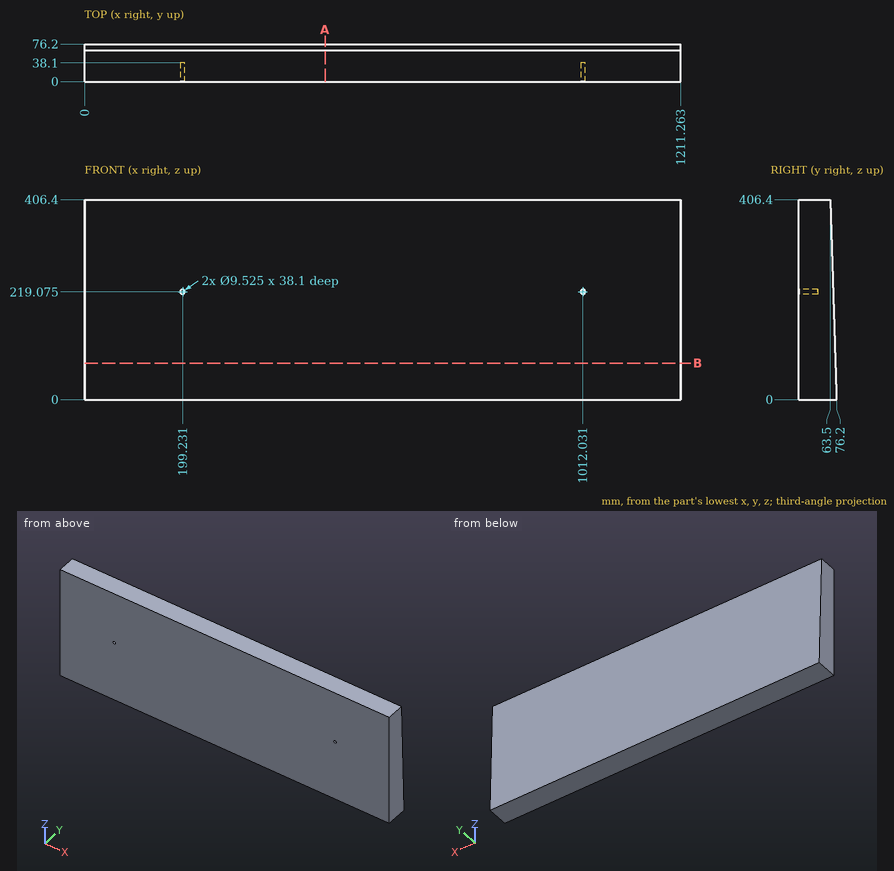
Drawing for the job (mm, zero at the part's lowest x, y, z). Give positions to 0.01 mm unless a question says otherwise; leave off trailing zeros. Loops run counter-clockwise (first coordinate to the right, second up) from the corner with the lowest first, then second, coordinate; pieces in that order, holes last.
Item 1: Drop flat-ended pins along their axis: P1, Ø6, axis at x = 156, z = 135.5, coming from the +Y side; P2, Ø3, axis at x = 517, z = 117.5, coming from the +Y side (1 decimal); P3, Ø3, axis at x = 199, z = 217, coming from the -Y side. Give the stop position or say it passes through.
Check values:
P1: stops at y = 72.06
P2: stops at y = 72.6
P3: stops at y = 38.1
Item 2: Drill centre lines: line 1 along X through (y, z) = (22, 222.5) (1 decimal); line 2 along X through (y, z) = (14.5, 217.5) (1 decimal); line 3 along Y through (x, z) = (1106.5, 380) (1 decimal). Where is each one in solid material? Low to high.
Check values:
line 1: x = 0 to 195.9, 202.5 to 1008.7, 1015.3 to 1211.3
line 2: x = 0 to 194.7, 203.7 to 1007.5, 1016.5 to 1211.3
line 3: y = 0 to 64.3
Item 3: Slice it at A-A (x = 488.5). Write the cut outline in (y, z), plus the area to 3 significant figures.
Check values:
outline: (0, 0) - (76.2, 0) - (63.5, 406.4) - (0, 406.4) - close
area: 28,400 mm2
Item 4: Slice it at B-B (z = 74). Write the cut outline in (x, y).
Check values:
outline: (0, 0) - (1211.26, 0) - (1211.26, 73.89) - (0, 73.89) - close
